from build123d import *

# Parameters (mm, degrees)
SKETCH1_R           = 76
BOSS_EXTRUDE1_DEPTH = 25.4
CUT_EXTRUDE4_DEPTH  = 13.462
SKETCH5_R           = 7.874
CUT_EXTRUDE5_DEPTH  = 20
SKETCH13_R          = 70
CUT_EXTRUDE9_DEPTH  = 7.5
CUT_EXTRUDE11_DEPTH = 1.27
SKETCH16_W          = 41.91
SKETCH16_H          = 10.16
CUT_EXTRUDE12_DEPTH = 1.016


with BuildPart() as part:
    # Sketch1 → Boss-Extrude1 (new body)
    with BuildSketch(Plane(origin=(0, 0, 0), x_dir=(1, 0, 0), z_dir=(0, 1, 0))):
        Circle(SKETCH1_R)
    extrude(amount=BOSS_EXTRUDE1_DEPTH)

    # Sketch2 → Cut-Extrude4 (cut)
    with BuildSketch(Plane(origin=(0, 25.4, 0), x_dir=(1, 0, 0), z_dir=(0, 1, 0))):
        with BuildLine():
            Line((-58.007955522, 54.61), (58.007955522, 54.61))
            ThreePointArc((58.007955522, 54.61), (112.617955522, 0), (58.007955522, -54.61))
            Line((58.007955522, -54.61), (-58.007955522, -54.61))
            ThreePointArc((-58.007955522, -54.61), (-112.617955522, 0), (-58.007955522, 54.61))
        make_face()
    extrude(amount=-CUT_EXTRUDE4_DEPTH, mode=Mode.SUBTRACT)

    # Sketch5 → Cut-Extrude5 (cut)
    with BuildSketch(Plane(origin=(0, 11.938, 0), x_dir=(1, 0, 0), z_dir=(0, 1, 0))):
        Circle(SKETCH5_R)
    extrude(amount=-CUT_EXTRUDE5_DEPTH, mode=Mode.SUBTRACT)

    # Sketch13 → Cut-Extrude9 (cut)
    with BuildSketch(Plane(origin=(0, 0, 0), x_dir=(-1, 0, 0), z_dir=(0, -1, 0))):
        Circle(SKETCH13_R)
    extrude(amount=-CUT_EXTRUDE9_DEPTH, mode=Mode.SUBTRACT)

    # Sketch15 → Cut-Extrude11 (cut)
    with BuildSketch(Plane(origin=(0, 11.938, 0), x_dir=(1, 0, 0), z_dir=(0, 1, 0))):
        with BuildLine():
            Line((76, -25.4), (-76, -25.4))
            ThreePointArc((-76, -25.4), (-101.4, 0), (-76, 25.4))
            Line((-76, 25.4), (76, 25.4))
            ThreePointArc((76, 25.4), (101.4, 0), (76, -25.4))
        make_face()
    extrude(amount=-CUT_EXTRUDE11_DEPTH, mode=Mode.SUBTRACT)

    # Sketch16 → Cut-Extrude12 (cut)
    with BuildSketch(Plane(origin=(0, 10.668, 0), x_dir=(1, 0, 0), z_dir=(0, 1, 0))):
        with Locations((-48.768, -13.97)):
            Rectangle(SKETCH16_W, SKETCH16_H)
        with Locations((-48.768, 13.97)):
            Rectangle(SKETCH16_W, SKETCH16_H)
        with Locations((48.768, -13.97)):
            Rectangle(SKETCH16_W, SKETCH16_H)
        with Locations((48.768, 13.97)):
            Rectangle(SKETCH16_W, SKETCH16_H)
    extrude(amount=-CUT_EXTRUDE12_DEPTH, mode=Mode.SUBTRACT)


solid = part.part
Can you work these out from the model? Positions are in its coordinate system, mm. A direction names the side the tool comes from. Coordinates: 2 decimals unless noted, no trailing zeros. Write each loop counter-clockwise with the first axis right and the second up, starting at its lowest first coordinate (ties: lowest second). Pieces come first, ordered by that corner, then holes. Notation, with made-up numbers: (46, 51) -> (65, 51) arc R13 ccw to (65, 63) -> close; hole circle Ø7 at (30, 27.25). An arc over 180 degrees is marked (long way). Write item = value, one per line.
(1) Imagine slicing it at D-D (y = 4.25). Please give me the cut outline in (x, z), and give its area (3 significant figures).
Verdict:
outline = circle Ø152 at (0, 0); hole circle Ø140 at (0, 0)
area = 2,750 mm^2
(2) On a 3-axis mill with a long thin cutter (end or side, diameter ignored), from which of +Z, -Z, +X, -X, +Y, -Y can I reach the whole of each face in a straight line? I mean faces 4 (the face through (-1.707, 9.106, 7.687)), 5 (the face through (55.55, 3.698, 42.594)), 6 (the face through (1, 10.668, -12)), 7 (the face through (-49, 9.652, -14)), 8 (the face through (-1, 25.4, -63)). Say none if no direction works.
Verdict:
face_4 = +Y, -Y
face_5 = -Y
face_6 = +X, -X, +Y
face_7 = +Y
face_8 = +Z, -Z, +X, -X, +Y
(3) Imagine slicing it at A-A (z = 0). Please give me the cut outline in (x, y).
Verdict:
outline = (-76, 0) -> (-70, 0) -> (-70, 7.5) -> (-7.87, 7.5) -> (-7.87, 10.67) -> (-76, 10.67) -> close; (7.87, 7.5) -> (70, 7.5) -> (70, 0) -> (76, 0) -> (76, 10.67) -> (7.87, 10.67) -> close
(4) Imagine slicing it at C-C (y = 16.75). Please give me the cut outline in (x, z).
Verdict:
outline = (-52.86, -54.61) arc R76 ccw to (52.86, -54.61) -> close; (-52.86, 54.61) -> (52.86, 54.61) arc R76 ccw to start
(5) If I drill on probe 1 along X at (y, z) = (9.4, 0); probe 2 along Z at (x, y) = (0, 4), over which ranges is the centre line in solid material (lowest first)?
Verdict:
probe_1 = -76 to -7.87, 7.87 to 76
probe_2 = -76 to -70, 70 to 76
(6) For pin 1 (18 mm diameter, centred on x = 0, z = 0, fed in from +Y); pin 2 (5 mm diameter, centred on x = 45, z = 13.5, fed in from +Y); pin 3 (0.8 mm diameter, centred on x = -40.5, y = 10.5, fed in from +Z), each with a flat end and sliding along its axis, tell me the tip position at first contact or that it passes through.
Verdict:
pin_1 = 10.67
pin_2 = 9.65
pin_3 = 64.56
(7) Thinking about a two-plate mould opening in X: for faces 1 (the face through (70.205, 9.7, 29.108)), 2 (the face through (-49, 9.652, 14)), 3 (the face through (-1, 25.4, 63)), which applies, +X half, -X half, draft (parallel to the pull), parting line (faces both ways), or undercut?
Verdict:
face_1 = parting line
face_2 = undercut
face_3 = draft
(8) Imagine slicing it at B-B (x = 0). Please give me the cut outline in (y, z).
Verdict:
outline = (0, -76) -> (25.4, -76) -> (25.4, -54.61) -> (11.94, -54.61) -> (11.94, -25.4) -> (10.67, -25.4) -> (10.67, -7.87) -> (7.5, -7.87) -> (7.5, -70) -> (0, -70) -> close; (0, 70) -> (7.5, 70) -> (7.5, 7.87) -> (10.67, 7.87) -> (10.67, 25.4) -> (11.94, 25.4) -> (11.94, 54.61) -> (25.4, 54.61) -> (25.4, 76) -> (0, 76) -> close
